```python
from build123d import *

# Parameters (mm, degrees)
ESQUISSE1_R          = 25
ESQUISSE1_R_2        = 6.5
BASE_EXTRUSION_DEPTH = 0.5


with BuildPart() as part:
    # Esquisse1 → Base-Extrusion (new body)
    with BuildSketch(Plane.XY):
        Circle(ESQUISSE1_R)
        Circle(ESQUISSE1_R_2, mode=Mode.SUBTRACT)
        with BuildLine():
            Line((15.627789901, -5.269931956), (17.438858637, -6.315552979))
            ThreePointArc((17.438858637, -6.315552979), (19.22097058, -6.424235968), (20.379791125, -5.065976084))
            ThreePointArc((20.379791125, -5.065976084), (20.979912421, 0.918299961), (19.85921918, 6.8272552))
            ThreePointArc((19.85921918, 6.8272552), (19.506948441, 7.307050839), (18.9444347, 7.501670519))
            ThreePointArc((18.9444347, 7.501670519), (16.02146997, 9.25), (15.96885459, 12.655526451))
            ThreePointArc((15.96885459, 12.655526451), (16.081565873, 13.239987481), (15.842186031, 13.784960709))
            ThreePointArc((15.842186031, 13.784960709), (11.285227305, 17.709987145), (5.802631579, 20.18240488))
            ThreePointArc((5.802631579, 20.18240488), (4.046933742, 19.857966791), (3.25, 18.260271082))
            Line((3.25, 18.260271082), (3.25, 16.169029037))
            ThreePointArc((3.25, 16.169029037), (3.632085584, 14.993293973), (4.632352941, 14.266790327))
            ThreePointArc((4.632352941, 14.266790327), (8.545219659, 12.327985276), (11.73385087, 9.344342875))
            ThreePointArc((11.73385087, 9.344342875), (11.875803373, 9.199177654), (12.044151428, 9.085677052))
            ThreePointArc((12.044151428, 9.085677052), (13.423393759, 7.75), (13.890502851, 5.887702578))
            ThreePointArc((13.890502851, 5.887702578), (13.904623229, 5.685158584), (13.959363746, 5.4896415))
            ThreePointArc((13.959363746, 5.4896415), (14.948958256, 1.236384668), (14.671579324, -3.121659837))
            ThreePointArc((14.671579324, -3.121659837), (14.800616259, -4.351168602), (15.627789901, -5.269931956))
        make_face(mode=Mode.SUBTRACT)
        with BuildLine():
            Line((-12.377789901, -10.899097081), (-14.188858637, -11.944718103))
            ThreePointArc((-14.188858637, -11.944718103), (-15.174036838, -13.433730824), (-14.577159546, -15.116428796))
            ThreePointArc((-14.577159546, -15.116428796), (-9.694685116, -18.628287106), (-4.017033149, -20.612215909))
            ThreePointArc((-4.017033149, -20.612215909), (-3.425382567, -20.547038319), (-2.97558011, -20.15719697))
            ThreePointArc((-2.97558011, -20.15719697), (0, -18.5), (2.97558011, -20.15719697))
            ThreePointArc((2.97558011, -20.15719697), (3.425382567, -20.547038319), (4.017033149, -20.612215909))
            ThreePointArc((4.017033149, -20.612215909), (9.694685116, -18.628287106), (14.577159546, -15.116428796))
            ThreePointArc((14.577159546, -15.116428796), (15.174036838, -13.433730824), (14.188858637, -11.944718103))
            Line((14.188858637, -11.944718103), (12.377789901, -10.899097081))
            ThreePointArc((12.377789901, -10.899097081), (11.168530675, -10.642125371), (10.039226383, -11.14513049))
            ThreePointArc((10.039226383, -11.14513049), (6.403738597, -13.564369944), (2.225512876, -14.833984375))
            ThreePointArc((2.225512876, -14.833984375), (2.028819856, -14.884336239), (1.846351423, -14.97337963))
            ThreePointArc((1.846351423, -14.97337963), (0, -15.5), (-1.846351423, -14.97337963))
            ThreePointArc((-1.846351423, -14.97337963), (-2.028819856, -14.884336239), (-2.225512876, -14.833984375))
            ThreePointArc((-2.225512876, -14.833984375), (-6.403738597, -13.564369944), (-10.039226383, -11.14513049))
            ThreePointArc((-10.039226383, -11.14513049), (-11.168530675, -10.642125371), (-12.377789901, -10.899097081))
        make_face(mode=Mode.SUBTRACT)
        with BuildLine():
            Line((-3.25, 16.169029037), (-3.25, 18.260271082))
            ThreePointArc((-3.25, 18.260271082), (-4.046933742, 19.857966791), (-5.802631579, 20.18240488))
            ThreePointArc((-5.802631579, 20.18240488), (-11.285227305, 17.709987145), (-15.842186031, 13.784960709))
            ThreePointArc((-15.842186031, 13.784960709), (-16.081565873, 13.239987481), (-15.96885459, 12.655526451))
            ThreePointArc((-15.96885459, 12.655526451), (-16.02146997, 9.25), (-18.9444347, 7.501670519))
            ThreePointArc((-18.9444347, 7.501670519), (-19.506948441, 7.307050839), (-19.85921918, 6.8272552))
            ThreePointArc((-19.85921918, 6.8272552), (-20.979912421, 0.918299961), (-20.379791125, -5.065976084))
            ThreePointArc((-20.379791125, -5.065976084), (-19.22097058, -6.424235968), (-17.438858637, -6.315552979))
            Line((-17.438858637, -6.315552979), (-15.627789901, -5.269931956))
            ThreePointArc((-15.627789901, -5.269931956), (-14.800616259, -4.351168602), (-14.671579324, -3.121659837))
            ThreePointArc((-14.671579324, -3.121659837), (-14.948958256, 1.236384668), (-13.959363746, 5.4896415))
            ThreePointArc((-13.959363746, 5.4896415), (-13.904623229, 5.685158584), (-13.890502851, 5.887702578))
            ThreePointArc((-13.890502851, 5.887702578), (-13.423393759, 7.75), (-12.044151428, 9.085677052))
            ThreePointArc((-12.044151428, 9.085677052), (-11.875803373, 9.199177654), (-11.73385087, 9.344342875))
            ThreePointArc((-11.73385087, 9.344342875), (-8.545219659, 12.327985276), (-4.632352941, 14.266790327))
            ThreePointArc((-4.632352941, 14.266790327), (-3.632085584, 14.993293973), (-3.25, 16.169029037))
        make_face(mode=Mode.SUBTRACT)
    extrude(amount=BASE_EXTRUSION_DEPTH)


solid = part.part
```
For this review, take the finished solid that the model builds, in its own axes (mm). Coordinates: 2 decimals unless noted, no trailing zeros. Write each loop counter-clockwise with the first axis right and the second up, starting at its lowest first coordinate (ties: lowest second). Pieces come first, ordered by that corner, then holes. Notation, with made-up numbers: (64.25, 15) - (106.25, 15) arc R15 ccw to (106.25, 32) - close; hole circle Ø1 at (11.5, 56.25). An arc over 180 degrees is marked (long way). Answer in a Markdown table with one row per item. Add a question column.
Q1. For P1, Ø10.5, axis at x = 0, y = 0, coming from the +Z side; P2, Ø5, axis at x = -6, y = 18.5, coming from the -Z side, all flat-tipped, find the tip position at first contact; note any pin that passes through.
Q2. For probe 1 along X at (y, z) = (9.5, 0.3); probe 2 along X at (y, z) = (9, 0.2); probe 3 along X at (y, z) = (2, 0.45), list the stretches that pass through material, from the lowest coordinate up.
Q3. We need section A-A, the plane y = 0. State the section outline as (x, z) points.
Q4. We need section D-D, the plane z = 0.15. Count the separate pieces of the cut face and the enclosed holes in it, and give its area (3 significant figures).
Q5. Draft analysis for pull direction Y (two halves, no side actions). For faces 1 (the cylindrical face through (3.62, 15.01, 0.25)), 2 (the cylindrical face through (23.846, 7.509, 0.246)), 3 (the flat face through (5, -5, 0)), state which applies: +Y half, -Y half, draft (parallel to the pull), parting line (faces both ways), or undercut.
Q6. We need section C-C, the plane y = 15.5. State the section outline as (x, z) points.
Q7. We need section B-B, the plane x = 0. State the section outline as (y, z) points, and give its area (3 significant figures).
Answer list:
| question | item | result |
|---|---|---|
| 1 | P1 | passes through |
| 1 | P2 | stops at z = 0 |
| 2 | probe 1 | x = -23.12 to -15.89, -11.61 to 11.61, 15.89 to 23.12 |
| 2 | probe 2 | x = -23.32 to -16.18, -12.2 to 12.2, 16.18 to 23.32 |
| 2 | probe 3 | x = -24.92 to -20.9, -14.87 to -6.18, 6.18 to 14.87, 20.9 to 24.92 |
| 3 | outline | (-25, 0) - (-21, 0) - (-21, 0.5) - (-25, 0.5) - close; (-15, 0) - (-6.5, 0) - (-6.5, 0.5) - (-15, 0.5) - close; (6.5, 0) - (15, 0) - (15, 0.5) - (6.5, 0.5) - close; (21, 0) - (25, 0) - (25, 0.5) - (21, 0.5) - close |
| 4 | separate pieces | 1 |
| 4 | enclosed holes | 4 |
| 4 | area | 1,320 mm2 |
| 5 | face 1 | undercut |
| 5 | face 2 | parting line |
| 5 | face 3 | draft |
| 6 | outline | (-19.62, 0) - (-14.17, 0) - (-14.17, 0.5) - (-19.62, 0.5) - close; (-3.37, 0) - (3.37, 0) - (3.37, 0.5) - (-3.37, 0.5) - close; (14.17, 0) - (19.62, 0) - (19.62, 0.5) - (14.17, 0.5) - close |
| 7 | outline | (-25, 0) - (-18.5, 0) - (-18.5, 0.5) - (-25, 0.5) - close; (-15.5, 0) - (-6.5, 0) - (-6.5, 0.5) - (-15.5, 0.5) - close; (6.5, 0) - (25, 0) - (25, 0.5) - (6.5, 0.5) - close |
| 7 | area | 17.0 mm2 |
